```python
from build123d import *

# Parameters (mm, degrees)
SKETCH1_W                      = 16
SKETCH1_H                      = 5
BASE_FLANGE1_DEPTH             = 1.2446
EDGE_FLANGE1_STRIP_W           = 6.9784
EDGE_FLANGE1_STRIP_H           = 1.2446
EDGE_FLANGE1_STRIP_CUT_DEPTH   = 5
EDGE_FLANGE1_STRIP_2_W         = 6.9784
EDGE_FLANGE1_STRIP_2_H         = 1.2446
EDGE_FLANGE1_STRIP_CUT_2_DEPTH = 5
EDGE_FLANGE1_DEPTH             = 5
EDGE_FLANGE1_BEND_DEPTH        = 5
EDGE_FLANGE2_STRIP_W           = 6.9784
EDGE_FLANGE2_STRIP_H           = 1.2446
EDGE_FLANGE2_STRIP_CUT_DEPTH   = 15.7554
EDGE_FLANGE2_STRIP_2_W         = 6.9784
EDGE_FLANGE2_STRIP_2_H         = 1.2446
EDGE_FLANGE2_STRIP_CUT_2_DEPTH = 15.7554
EDGE_FLANGE2_DEPTH             = 15.7554
EDGE_FLANGE2_BEND_DEPTH        = 15.7554
SKETCH15_R                     = 6
CUT_EXTRUDE1_DEPTH             = 20.778929656
SKETCH16_W                     = 11.1125
SKETCH16_H                     = 1
CUT_EXTRUDE2_DEPTH             = 26.231249968
SKETCH17_W                     = 18.4892
SKETCH17_H                     = 1
CUT_EXTRUDE3_DEPTH             = 21.129607236


# Sheet-metal steps are written as plain solids
with BuildPart() as part:
    # Sketch1 → Base-Flange1 (new body)
    with BuildSketch(Plane.XY):
        Rectangle(SKETCH1_W, SKETCH1_H)
    extrude(amount=-BASE_FLANGE1_DEPTH)

    # Edge-Flange1 strip (across the edge) → Edge-Flange1 strip cut (cut)
    with BuildSketch(Plane(origin=(8, -2.5, 0), x_dir=(-1, 0, 0), z_dir=(0, 1, 0))):
        with Locations((-2.4892, -0.6223)):
            Rectangle(EDGE_FLANGE1_STRIP_W, EDGE_FLANGE1_STRIP_H)
    extrude(amount=EDGE_FLANGE1_STRIP_CUT_DEPTH, mode=Mode.SUBTRACT)

    # Edge-Flange1 strip 2 (across the edge) → Edge-Flange1 strip cut 2 (cut)
    with BuildSketch(Plane(origin=(-8, 2.5, 0), x_dir=(1, 0, 0), z_dir=(0, -1, 0))):
        with Locations((-2.4892, -0.6223)):
            Rectangle(EDGE_FLANGE1_STRIP_2_W, EDGE_FLANGE1_STRIP_2_H)
    extrude(amount=EDGE_FLANGE1_STRIP_CUT_2_DEPTH, mode=Mode.SUBTRACT)

    # Edge-Flange1 section (across the edge) → Edge-Flange1 (add)
    with BuildSketch(Plane(origin=(8, -2.5, 0), x_dir=(-1, 0, 0), z_dir=(0, 1, 0))):
        with BuildLine():
            Line((-1.2446, 1), (-1.2446, 16.7554))
            Line((-1.2446, 16.7554), (0, 16.7554))
            Line((0, 16.7554), (0, 1))
            ThreePointArc((0, 1), (0.292893219, 0.292893219), (1, 0))
            Line((1, 0), (1, -1.2446))
            ThreePointArc((1, -1.2446), (-0.587171881, -0.587171881), (-1.2446, 1))
        make_face()
    extrude(amount=EDGE_FLANGE1_DEPTH)

    # Edge-Flange1 section 2 (across the edge) → Edge-Flange1 bend (add)
    with BuildSketch(Plane(origin=(-8, 2.5, 0), x_dir=(1, 0, 0), z_dir=(0, -1, 0))):
        with BuildLine():
            Line((-1.2446, 1), (-1.2446, 16.7554))
            Line((-1.2446, 16.7554), (0, 16.7554))
            Line((0, 16.7554), (0, 1))
            ThreePointArc((0, 1), (0.292893219, 0.292893219), (1, 0))
            Line((1, 0), (1, -1.2446))
            ThreePointArc((1, -1.2446), (-0.587171881, -0.587171881), (-1.2446, 1))
        make_face()
    extrude(amount=EDGE_FLANGE1_BEND_DEPTH)

    # Edge-Flange2 strip (across the edge) → Edge-Flange2 strip cut (cut)
    with BuildSketch(Plane(origin=(-8, -2.5, 16.7554), x_dir=(0, 1, 0), z_dir=(0, 0, -1))):
        with Locations((-2.4892, -0.6223)):
            Rectangle(EDGE_FLANGE2_STRIP_W, EDGE_FLANGE2_STRIP_H)
    extrude(amount=EDGE_FLANGE2_STRIP_CUT_DEPTH, mode=Mode.SUBTRACT)

    # Edge-Flange2 strip 2 (across the edge) → Edge-Flange2 strip cut 2 (cut)
    with BuildSketch(Plane(origin=(8, -2.5, 1), x_dir=(0, 1, 0), z_dir=(0, 0, 1))):
        with Locations((-2.4892, -0.6223)):
            Rectangle(EDGE_FLANGE2_STRIP_2_W, EDGE_FLANGE2_STRIP_2_H)
    extrude(amount=EDGE_FLANGE2_STRIP_CUT_2_DEPTH, mode=Mode.SUBTRACT)

    # Edge-Flange2 section (across the edge) → Edge-Flange2 (add)
    with BuildSketch(Plane(origin=(-8, -2.5, 16.7554), x_dir=(0, 1, 0), z_dir=(0, 0, -1))):
        with BuildLine():
            Line((-1.2446, 1), (-1.2446, 6.1214))
            Line((-1.2446, 6.1214), (0, 6.1214))
            Line((0, 6.1214), (0, 1))
            ThreePointArc((0, 1), (0.292893219, 0.292893219), (1, 0))
            Line((1, 0), (1, -1.2446))
            ThreePointArc((1, -1.2446), (-0.587171881, -0.587171881), (-1.2446, 1))
        make_face()
    extrude(amount=EDGE_FLANGE2_DEPTH)

    # Edge-Flange2 section 2 (across the edge) → Edge-Flange2 bend (add)
    with BuildSketch(Plane(origin=(8, -2.5, 1), x_dir=(0, 1, 0), z_dir=(0, 0, 1))):
        with BuildLine():
            Line((-1.2446, 1), (-1.2446, 6.1214))
            Line((-1.2446, 6.1214), (0, 6.1214))
            Line((0, 6.1214), (0, 1))
            ThreePointArc((0, 1), (0.292893219, 0.292893219), (1, 0))
            Line((1, 0), (1, -1.2446))
            ThreePointArc((1, -1.2446), (-0.587171881, -0.587171881), (-1.2446, 1))
        make_face()
    extrude(amount=EDGE_FLANGE2_BEND_DEPTH)

    # Sketch15 → Cut-Extrude1 (cut, through all)
    with BuildSketch(Plane(origin=(0, -2.5, 0), x_dir=(1, 0, 0), z_dir=(0, 1, 0))):
        with Locations((0, -8.8777)):
            Circle(SKETCH15_R)
    extrude(amount=-CUT_EXTRUDE1_DEPTH, mode=Mode.SUBTRACT)

    # Sketch16 → Cut-Extrude2 (cut, through all)
    with BuildSketch(Plane(origin=(9.2446, 0, 0), x_dir=(0, 0, -1), z_dir=(1, 0, 0))):
        with Locations((-8.8777, 0.5)):
            Rectangle(SKETCH16_W, SKETCH16_H)
    extrude(amount=-CUT_EXTRUDE2_DEPTH, mode=Mode.SUBTRACT)

    # Sketch17 → Cut-Extrude3 (cut, through all)
    with BuildSketch(Plane(origin=(0, 2.5, 0), x_dir=(1, 0, 0), z_dir=(0, 1, 0))):
        with Locations((0, -16.2554)):
            Rectangle(SKETCH17_W, SKETCH17_H)
    extrude(amount=-CUT_EXTRUDE3_DEPTH, mode=Mode.SUBTRACT)


solid = part.part
```
Model file for the job. Use its own axes, mm. A direction names the side the tool comes from. Coordinates: 2 decimals unless noted, no trailing zeros. Loops run counter-clockwise (first coordinate to the right, second up) from the corner with the lowest first, then second, coordinate; pieces in that order, holes last. Notation, with made-up numbers: (89.5, -34) - (132.5, -34) arc R26 ccw to (132.5, -5) - close; hole circle Ø8 at (-16, -26). An arc over 180 degrees is marked (long way). Write item = value, one per line. Start each with the question number.
Item 1: Saw through at D-D, the plane z = 14. List the corners of the cut face in (x, y), then the cut area to 3 significant figures.
Item 2: Pull direction Z, two halves, no side cores. Call faces 4 (the face through (0, 0, -1.245)), 5 (the face through (0.1, -2.5, -0.4)), 6 (the face through (6, -3, 9)), 7 (the face through (8.6, 0.5, 14.434)): +Z half, -Z half, draft (parallel to the pull), parting line (faces both ways), or undercut.
Item 3: Wall check: probe 1 along X at (y, z) = (2, 6); probe 2 along Z at (x, y) = (0.75, 1.75); probe 3 along X at (y, z) = (-3, 6). Give the ranges that are in metal, low to high. Write a range as [from, to].
Item 4: Saw through at A-A, the plane z = 1.75. List the corners of the cut face in (x, y).
Item 5: Saw through at C-C, the plane x = 7.25. List the corners of the cut face in (y, z), then the cut area to 3 significant figures.
Item 6: Saw through at B-B, the plane y = 0.25. List the corners of the cut face in (x, z).
Item 7: Drop flat-ended pins along their axis: pin 1 Ø1.3 at (y, z) = (-3, 15) entering from +X; pin 2 Ø8 at (x, z) = (3, 2) entering from +Y; pin 3 Ø1.5 at (x, z) = (3.5, 9.5) entering from +Y; pin 4 Ø1 at (y, z) = (-3, 1.5) entering from -X. Give the stop position or say it passes through.
Item 8: 3-axis set-ups, long thin cutter, end or side, ignore diameter. For faces 1 (the face through (8.6, 0.5, 3.321)), 2 (the face through (8.605, -3.07, 8.274)), 3 (the face through (0, 0, 0)): which of +Z, -Z, +X, -X, +Y, -Y reach the whole face in a straight line?
Answers:
q1.outline = (-9.24, -1.5) arc R2.24 ccw to (-7, -3.74) - (-3.12, -3.74) - (-3.12, -2.5) - (-7, -2.5) arc R1 cw to (-8, -1.5) - (-8, 0) - (-9.24, 0) - close; (-9.24, 1) - (-8, 1) - (-8, 2.5) - (-9.24, 2.5) - close; (3.12, -3.74) - (7, -3.74) arc R2.24 ccw to (9.24, -1.5) - (9.24, 0) - (8, 0) - (8, -1.5) arc R1 cw to (7, -2.5) - (3.12, -2.5) - close; (8, 1) - (9.24, 1) - (9.24, 2.5) - (8, 2.5) - close
q1.area = 23.5 mm2
q2.face_4 = -Z half
q2.face_5 = draft
q2.face_6 = undercut
q2.face_7 = undercut
q3.probe_1 = [-9.24, -8], [8, 9.24]
q3.probe_2 = [-1.24, 0]
q3.probe_3 = [-8.67, -5.26], [5.26, 8.67]
q4.outline = (-9.24, -1.5) arc R2.24 ccw to (-7, -3.74) - (-1.88, -3.74) - (-1.88, -2.5) - (-7, -2.5) arc R1 cw to (-8, -1.5) - (-8, 2.5) - (-9.24, 2.5) - close; (1.88, -3.74) - (7, -3.74) arc R2.24 ccw to (9.24, -1.5) - (9.24, 2.5) - (8, 2.5) - (8, -1.5) arc R1 cw to (7, -2.5) - (1.88, -2.5) - close
q5.outline = (-3.73, 1) - (-2.47, 1) - (-2.47, 15.76) - (-3.73, 15.76) - close; (-2.5, -1.23) - (2.5, -1.23) - (2.5, 0.03) - (-2.5, 0.03) - close
q5.area = 24.9 mm2
q6.outline = (-9.24, 1) arc R2.24 ccw to (-7, -1.24) - (7, -1.24) arc R2.24 ccw to (9.24, 1) - (9.24, 3.32) - (8, 3.32) - (8, 1) arc R1 cw to (7, 0) - (-7, 0) arc R1 cw to (-8, 1) - (-8, 3.32) - (-9.24, 3.32) - close; (-9.24, 14.43) - (-8, 14.43) - (-8, 15.76) - (-9.24, 15.76) - close; (8, 14.43) - (9.24, 14.43) - (9.24, 15.76) - (8, 15.76) - close
q7.pin_1 = 9.08
q7.pin_2 = 2.5
q7.pin_3 = through
q7.pin_4 = -9.01
q8.face_1 = +X, -X
q8.face_2 = +Z, +X, -Y
q8.face_3 = +Z, +Y, -Y
